CAD build for the part. Positions are in the model's coordinates, mm. Face numbers are marked on the shaded views. A direction names the side the tool comes from. Give positions to 0.01 mm unless a question says otherwise; leave off trailing zeros. Loops run counter-clockwise (first coordinate to the right, second up) from the corner with the lowest first, then second, coordinate; pieces in that order, holes last.
Item 1: Saw through at C-C on z = -3. Give the cut face in (x, y), plus the area to 3 significant figures.
Item 2: Mould opens along Z. For the marked faces 1, 2, 3 and 4 say: released by +Z, released by -Z, zero draft, split by the parting line, or undercut.
Item 3: Probe probe 1 along X at (y, z) = (91, 0); probe 2 along X at (y, z) = (77.5, 35). List the from-to ranges inside material, lowest first.
Item 4: Saw through at B-B on x = 28. Give the cut face in (y, z).
Item 5: Saw through at D-D on z = -39. Give the cut face in (x, y).
Item 6: Which spindle directions (+Z, -Z, +X, -X, +Y, -Y) get a long thin tool onto all of the face, cutting with end or side? Do the marked faces 5, 6, 7, 8 and 9. Say none if no direction does.
Item 7: Saw through at A-A on y = 46. Give the cut face in (x, z).
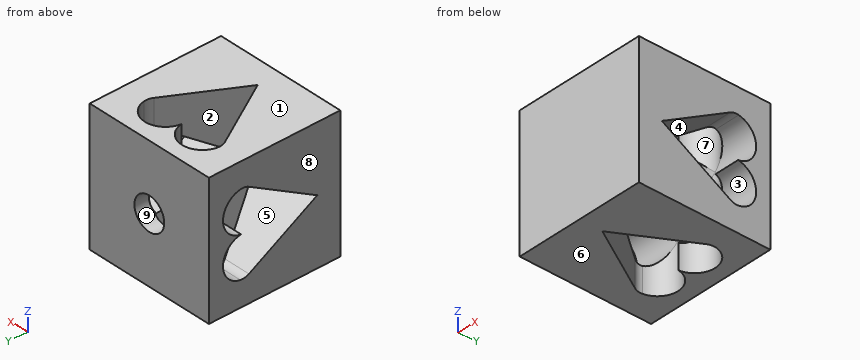
from build123d import *

# Parameters (mm, degrees)
SKETCH1_W           = 100
SKETCH1_H           = 100
BOSS_EXTRUDE1_DEPTH = 100
CUT_EXTRUDE1_DEPTH  = 50
CIRPATTERN2_COUNT   = 4
SKETCH3_R           = 12.5
CUT_EXTRUDE2_DEPTH  = 50


with BuildPart() as part:
    # Sketch1 → Boss-Extrude1 (new body)
    with BuildSketch(Plane(origin=(0, 0, 0), x_dir=(1, 0, 0), z_dir=(0, 1, 0))):
        Rectangle(SKETCH1_W, SKETCH1_H)
    extrude(amount=BOSS_EXTRUDE1_DEPTH)

    # Sketch2 → Cut-Extrude1 (cut)
    with BuildSketch(Plane.XY.offset(50)):
        with BuildLine():
            Line((0, 17.495781671), (-29.788286543, 69.516301586))
            ThreePointArc((-29.788286543, 69.516301586), (-30.943422674, 72.666080294), (-30.99180085, 76.020645087))
            ThreePointArc((-30.99180085, 76.020645087), (-15.265826761, 89.261609896), (0, 75.492661373))
            ThreePointArc((0, 75.492661373), (15.265826761, 89.261609896), (30.99180085, 76.020645087))
            ThreePointArc((30.99180085, 76.020645087), (30.943422674, 72.666080294), (29.788286543, 69.516301586))
            Line((29.788286543, 69.516301586), (0, 17.495781671))
        make_face()
    cut_extrude1 = extrude(amount=-CUT_EXTRUDE1_DEPTH, mode=Mode.SUBTRACT)

    # CirPattern2: Cut-Extrude1 ×4 about axis
    cirpattern2_axis = Axis((0, 0, 0), (0, 1, 0))
    for i in range(1, CIRPATTERN2_COUNT):
        add(cut_extrude1.rotate(cirpattern2_axis, i * 360 / CIRPATTERN2_COUNT), mode=Mode.SUBTRACT)

    # Sketch3 → Cut-Extrude2 (cut)
    with BuildSketch(Plane(origin=(0, 100, 0), x_dir=(1, 0, 0), z_dir=(0, 1, 0))):
        with Locations(Location((0, 0, 0), (0, 0, 270))):
            Circle(SKETCH3_R)
    extrude(amount=-CUT_EXTRUDE2_DEPTH, mode=Mode.SUBTRACT)


solid = part.part
Results below:
1. outline: (-50, 0) - (50, 0) - (50, 22.73) - (3, 22.73) - (0, 17.5) - (-3, 22.73) - (-50, 22.73) - close; (-50, 82.98) - (-28.06, 82.98) arc R15.64 cw to (-12.13, 88.89) - (-12.13, 100) - (-50, 100) - close; (12.13, 88.89) arc R15.64 cw to (28.06, 82.98) - (50, 82.98) - (50, 100) - (12.13, 100) - close
1. area: 3,390 mm2
2. face 1: released by +Z
2. face 2: zero draft
2. face 3: undercut
2. face 4: undercut
3. probe 1: x = -50 to -12.5, 12.5 to 50
3. probe 2: x = -50 to -30.69, -0.38 to 0.38, 30.69 to 50
4. outline: (0, -50) - (66.39, -50) - (66.39, -28) - (17.5, 0) - (66.39, 28) - (66.39, 50) - (0, 50) - close; (83.07, -50) - (100, -50) - (100, 50) - (83.07, 50) - (83.07, 28) arc R15.64 cw to (83.07, 3.06) - (83.07, -3.06) arc R15.64 cw to (83.07, -28) - close
5. outline: (-50, 0) - (50, 0) - (50, 100) - (-50, 100) - close; hole (-30.99, 76.02) arc R10 ccw to (-29.79, 69.52) - (0, 17.5) - (29.79, 69.52) arc R10 ccw to (30.99, 76.02) arc R15.64 ccw to (0, 75.49) arc R15.64 ccw to start
6. face 5: +X, -X
6. face 6: -Z, +X, -X, +Y, -Y
6. face 7: +Z, -Z
6. face 8: +Z, -Z, -X, +Y, -Y
6. face 9: +Y
7. outline: (-50, -50) - (-16.32, -50) - (-16.32, -16.32) - (-50, -16.32) - close; (-50, 16.32) - (-16.32, 16.32) - (-16.32, 50) - (-50, 50) - close; (16.32, -50) - (50, -50) - (50, -16.32) - (16.32, -16.32) - close; (16.32, 16.32) - (50, 16.32) - (50, 50) - (16.32, 50) - close
